Geometry check sheet. Reference: the model listing, model coordinates, mm. A direction names the side the tool comes from. Round coordinates to 2 decimals unless told otherwise and drop trailing zeros. Order: outer loops, then holes, each group sorted by start corner. A loop starts at its lowest first (then second) coordinate and runs counter-clockwise, first axis right, second up.
```python
from build123d import *

# Parameters (mm, degrees)
F2_SIZE  = 0.5
F3_R     = 1
F5_DEPTH = 3


with BuildPart() as f1:
    # F0 (on Front) → F1 (revolve)
    with BuildSketch(Plane.XZ):
        Polygon((-3, 0), (0, 0), (0, 31), (-5, 31), (-5, 25), (-3, 25), align=None)
    revolve(axis=Axis((0, 0, 15.604191), (0, 0, 1)))

    # F2
    f2_edges = [f1.edges().sort_by_distance(p)[0] for p in [
        (3, 0, 0),
    ]]
    chamfer(f2_edges, length=F2_SIZE)

    # F3
    f3_edges = [f1.edges().sort_by_distance(p)[0] for p in [
        (5, 0, 31),
    ]]
    fillet(f3_edges, radius=F3_R)

    # F4 (on face) → F5 (cut)
    with BuildSketch(Plane.XY.offset(31)):
        Polygon((-2, 1.154701), (-2, -1.154701), (0, -2.309401), (2, -1.154701), (2, 1.154701), (0, 2.309401), align=None)
    extrude(amount=-F5_DEPTH, mode=Mode.SUBTRACT)


solid = f1.part
```
(1) Material ranges on line 1 (Z direction, x = 0, y = -3.75); line 2 (Z direction, x = -1.25, y = 1); line 3 (Y direction, x = -1.25, z = 29), recorded low to high.
Returned:
line 1: z = 25 to 31
line 2: z = 0 to 28
line 3: y = -4.84 to -1.59, 1.59 to 4.84
(2) Sectioned sample at B-B, the plane z = 17. Record the cut outline in (x, y), and give its area (3 significant figures).
Returned:
outline: circle Ø6 at (0, 0)
area: 28.3 mm2
(3) Sectioned sample at A-A, the plane y = 0. Record the cut outline in (x, z), and give its area (3 significant figures).
Returned:
outline: (-5, 25) - (-3, 25) - (-3, 0.5) - (-2.5, 0) - (2.5, 0) - (3, 0.5) - (3, 25) - (5, 25) - (5, 30) arc R1 ccw to (4, 31) - (2, 31) - (2, 28) - (-2, 28) - (-2, 31) - (-4, 31) arc R1 ccw to (-5, 30) - close
area: 197 mm2
(4) Set-up check for faces 1 (the flat face through (0.99, -1.74, 29.52)), 2 (the flat face through (1, -2, 31)): record each of +Z, -Z, +X, -X, +Y, -Y from which the full face is reachable in a straight line by a thin tool's end or side.
Returned:
face 1: +Z
face 2: +Z, +X, -X, +Y, -Y
(5) Draft check along X on faces 3 (the cylindrical face through (3, 0, 13)), 4 (the flat face through (-3.3, -0.1, 25)), 5 (the flat face through (-2, 0, 30)). Enter one of: released by +X, released by -X, zero draft, split by the parting line, or undercut.
Returned:
face 3: split by the parting line
face 4: zero draft
face 5: undercut
(6) Depth check by flat-ended pin: P1, Ø4, axis at x = -3.5, z = 3.5, coming from the -Y side; P2, Ø1, axis at x = -1, z = 8, coming from the -Y side; P3, Ø3, axis at x = 0, y = 0.5, coming from the +Z side. Enter the tip coordinate at first touch or a pass-through.
Returned:
P1: stops at y = -2.6
P2: stops at y = -2.96
P3: stops at z = 28
